The listing builds one solid part. Answer for the finished solid, in the listing's coordinates (mm). Face numbers are marked on the shaded views. A direction names the side the tool comes from. Round coordinates to 2 decimals unless told otherwise and drop trailing zeros. Write each loop counter-clockwise with the first axis right and the second up, starting at its lowest first coordinate (ties: lowest second). Pieces come first, ordered by that corner, then holes.
(1) A cutting plane is placed at B-B, the plane z = 4.5. Give the vertices of the cut face in (x, y), and give its area (3 significant figures).
(2) A cutting plane is placed at C-C, the plane z = 46. Give the vertices of the cut face in (x, y).
(3) A cutting plane is placed at D-D, the plane y = -1.5. Give the number of separate pieces and of enclosed holes in the cut face, and give its area (3 significant figures).
(4) A cutting plane is placed at A-A, the plane x = 100.5. Give the vertices of the cut face in (y, z).
(5) Find the intervals of material crossed by probe 1 along X at (y, z) = (-3.75, 53.5); probe 2 along X at (y, z) = (1.5, 5.5); probe 3 along Z at (x, y) = (81.25, 0), in increasing order.
(6) Each of these flat-tipped pins is pushed along its axis until it touches: pin 1 Ø7.5 at (x, y) = (58.5, 5) entering from +Z; pin 2 Ø15 at (y, z) = (0, 46) entering from -X; pin 3 Ø8 at (x, y) = (65, -2) entering from -Z; pin 4 Ø6.5 at (x, y) = (100.5, 0) entering from -Z. Where does it stop, or does it pass through?
(7) The mould has two halves that part along X. Classify the marked faces 6, 7 and 8: +X half, -X half, draft (parallel to the pull), parting line (faces both ways), or undercut.
(8) For the marked faces 1, 2, 3, 4 and 5, determine the directions among +Z, -Z, +X, -X, +Y, -Y from which every point of the face is accessible in a straight line to the end or side of a thin tool.
from build123d import *

# Parameters (mm, degrees)
F0_W     = 10
F0_H     = 13
F1_DEPTH = 13
F2_R     = 5.5
F3_DEPTH = 13.001
F4_R     = 5.5
F5_DEPTH = 13.001
F6_R     = 6.5
F7_DEPTH = 88.001
F8_DEPTH = 88.001


with BuildPart() as f1:
    # F0 (on Front) → F1 (new body, symmetric)
    with BuildSketch(Plane.XZ):
        with Locations((5, 6.5)):
            Rectangle(F0_W, F0_H)
        Polygon((10, 13), (10, 0), (39, 0), (39, 17), (74, 17), (74, 0), (103, 0), (103, 13), (88, 13), (88, 64), (69, 64), (69, 30), (44, 30), (44, 64), (25, 64), (25, 13), align=None)
        with Locations((108, 6.5)):
            Rectangle(F0_W, F0_H)
    extrude(amount=F1_DEPTH, both=True)

    # F2 (on face) → F3 (cut, through all)
    with BuildSketch(Plane.XY.offset(13)):
        Polygon((0, -13), (10, -13), (0, -3), align=None)
        with Locations((12.5, 0)):
            Circle(F2_R)
    extrude(amount=-F3_DEPTH, mode=Mode.SUBTRACT)

    # F4 (on face) → F5 (cut, through all)
    with BuildSketch(Plane.XY.offset(13)):
        with Locations((100.5, 0)):
            Circle(F4_R)
        Polygon((113, -3), (103, -13), (113, -13), align=None)
    extrude(amount=-F5_DEPTH, mode=Mode.SUBTRACT)

    # F6 (on face) → F7 (cut, through all)
    with BuildSketch(Plane.YZ.offset(88)):
        with Locations((0, 46)):
            Circle(F6_R)
    extrude(amount=-F7_DEPTH, mode=Mode.SUBTRACT)

    # F6 (on face) → F8 (cut, through all)
    with BuildSketch(Plane.YZ.offset(88)):
        with BuildLine():
            Line((13, 64), (0, 64))
            ThreePointArc((0, 64), (6.619465, 63.368338), (13, 61.496154))
            Line((13, 61.496154), (13, 64))
        make_face()
        with BuildLine():
            ThreePointArc((-13, 61.496154), (-6.619465, 63.368338), (0, 64))
            Line((0, 64), (-13, 64))
            Line((-13, 64), (-13, 61.496154))
        make_face()
    extrude(amount=-F8_DEPTH, mode=Mode.SUBTRACT)


solid = f1.part
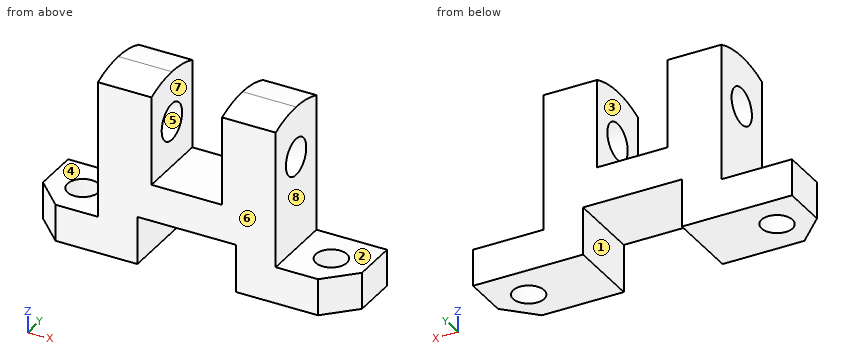
Solutions:
1. outline: (0, -3) - (10, -13) - (39, -13) - (39, 13) - (0, 13) - close; (74, -13) - (103, -13) - (113, -3) - (113, 13) - (74, 13) - close; hole circle Ø11 at (12.5, 0); hole circle Ø11 at (100.5, 0)
1. area: 1,740 mm2
2. outline: (25, -13) - (44, -13) - (44, -6.5) - (25, -6.5) - close; (25, 6.5) - (44, 6.5) - (44, 13) - (25, 13) - close; (69, -13) - (88, -13) - (88, -6.5) - (69, -6.5) - close; (69, 6.5) - (88, 6.5) - (88, 13) - (69, 13) - close
3. separate pieces: 5
3. enclosed holes: 0
3. area: 2,480 mm2
4. outline: (-13, 0) - (-5.5, 0) - (-5.5, 13) - (-13, 13) - close; (5.5, 0) - (13, 0) - (13, 13) - (5.5, 13) - close
5. probe 1: x = 25 to 44, 69 to 88
5. probe 2: x = 0 to 7.21, 17.79 to 39, 74 to 95.21, 105.79 to 113
5. probe 3: z = 0 to 39.5, 52.5 to 64
6. pin 1: stops at z = 30
6. pin 2: stops at x = 25
6. pin 3: stops at z = 17
6. pin 4: passes through
7. face 6: draft
7. face 7: undercut
7. face 8: +X half
8. face 1: -Z, +Y, -Y
8. face 2: +Z, +X, +Y, -Y
8. face 3: +Z, +Y, -Y
8. face 4: +Z, -X, +Y, -Y
8. face 5: +X, -X
